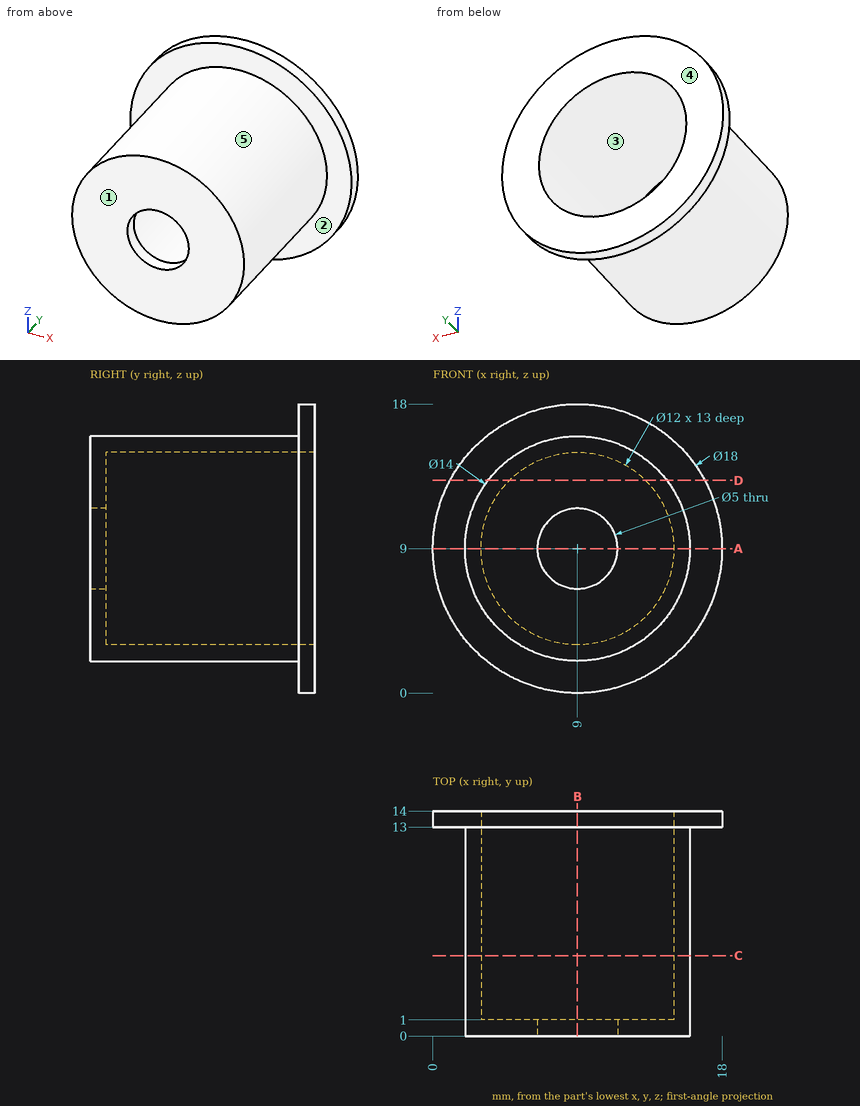
Design review of the part shown in the three views and the two pictorial views. Dimensions are in mm from the part's minimum x, y and z. A direction names the side the tool comes from. Round coordinates to 2 decimals unless told otherwise and drop trailing zeros. Order: outer loops, then holes, each group sorted by start corner. A loop starts at its lowest first (then second) coordinate and runs counter-clockwise, first axis right, second up.
Item 1: To check wall thickness, follow probe 1 along X at (y, z) = (0.2, 9); probe 2 along X at (y, z) = (10.5, 9); probe 3 along Y at (x, z) = (9.25, 5.25). State the ranges of each line that lie inside material, in increasing order.
Working result:
probe 1: x = 2 to 6.5, 11.5 to 16
probe 2: x = 2 to 3, 15 to 16
probe 3: y = 0 to 1
Item 2: Add section B-B, the plane x = 9. State the section outline as (y, z) points.
Working result:
outline: (0, 2) - (13, 2) - (13, 0) - (14, 0) - (14, 3) - (1, 3) - (1, 6.5) - (0, 6.5) - close; (0, 11.5) - (1, 11.5) - (1, 15) - (14, 15) - (14, 18) - (13, 18) - (13, 16) - (0, 16) - close
Item 3: Add section A-A, the plane z = 9. State the section outline as (x, y) points.
Working result:
outline: (0, 13) - (2, 13) - (2, 0) - (6.5, 0) - (6.5, 1) - (3, 1) - (3, 14) - (0, 14) - close; (11.5, 0) - (16, 0) - (16, 13) - (18, 13) - (18, 14) - (15, 14) - (15, 1) - (11.5, 1) - close
Item 4: Add section C-C, the plane y = 5. State the section outline as (x, z) points, and give its area (3 significant figures).
Working result:
outline: circle Ø14 at (9, 9); hole circle Ø12 at (9, 9)
area: 40.8 mm2
Item 5: Add section D-D, the plane z = 13.25. State the section outline as (x, y) points, and give its area (3 significant figures).
Working result:
outline: (1.07, 13) - (3.44, 13) - (3.44, 0) - (14.56, 0) - (14.56, 13) - (16.93, 13) - (16.93, 14) - (13.24, 14) - (13.24, 1) - (4.76, 1) - (4.76, 14) - (1.07, 14) - close
area: 50.4 mm2
Item 6: For pin 1 (2 mm diameter, centred on x = 9, y = 4, fed in from +Z); pin 2 (5 mm diameter, centred on x = 15.5, y = 11, fed in from -Z); pin 3 (1.5 mm diameter, centred on x = 12.5, z = 8.5, fed in from +Y), all flat-tipped, find the tip position at first contact; note any pin that passes through.
Working result:
pin 1: stops at z = 16
pin 2: stops at z = 1.52
pin 3: stops at y = 1
Item 7: Machinability: for the marked faces 1 and 2, which of the approach directions +Z, -Z, +X, -X, +Y, -Y give a long, thin tool a straight path to every point of the face, cutting with its end or side? Answer none if there is none.
Working result:
face 1: +Z, -Z, +X, -X, -Y
face 2: -Y
Item 8: Draft analysis for pull direction X (two halves, no side actions). For the marked faces 3, 4 and 5, state which applies: released by +X, released by -X, zero draft, split by the parting line, or undercut.
Working result:
face 3: undercut
face 4: zero draft
face 5: split by the parting line
